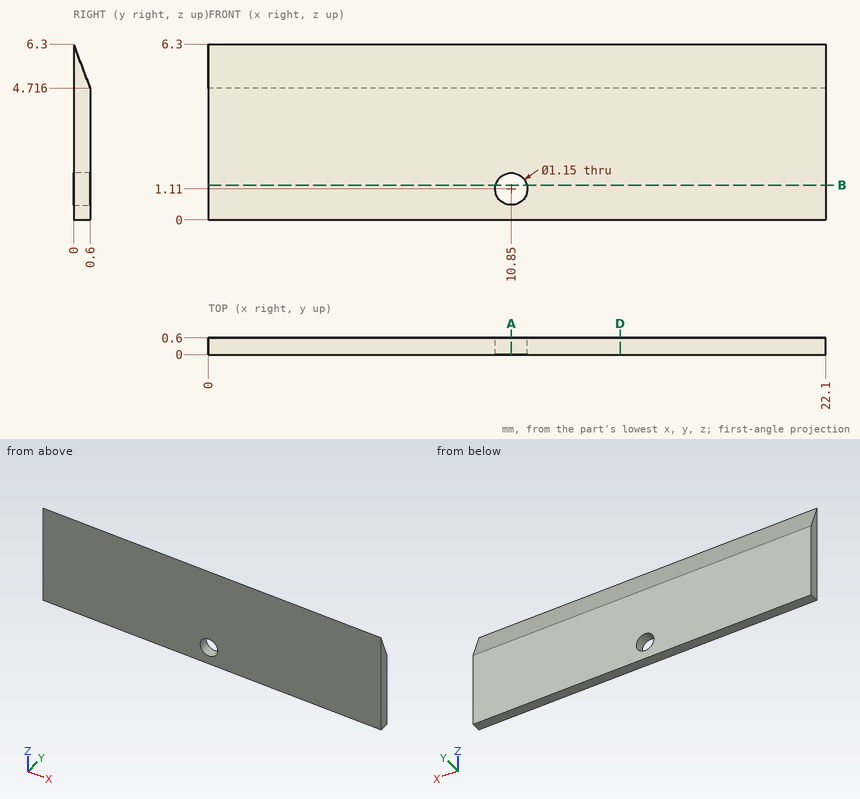
The drawing under review shows one solid part. Ordinate dimensions are in mm from its lowest x, y, z. Round coordinates to 2 decimals unless told otherwise and drop trailing zeros. Loops run counter-clockwise (first coordinate to the right, second up) from the corner with the lowest first, then second, coordinate; pieces in that order, holes last. Notation, with made-up numbers: (-16, 45) - (1, 45) arc R25 cw to (1, 64) - close; hole circle Ø9 at (79, 1.25). An arc over 180 degrees is marked (long way). One line per question, with ' | ' between items.
Q1. Take a section at D-D (x = 14.75). Give the boundary of the cut face in (y, z) (1 decimal).
Taken from the geometry:
outline: (0, 0) - (0.6, 0) - (0.6, 4.7) - (0, 6.3) - close
Q2. Take a section at A-A (x = 10.85). Give the boundary of the cut face in (y, z) (1 decimal).
Taken from the geometry:
outline: (0, 0) - (0.6, 0) - (0.6, 0.5) - (0, 0.5) - close; (0, 1.7) - (0.6, 1.7) - (0.6, 4.7) - (0, 6.3) - close
Q3. For line 1 along X through (y, z) = (0.1, 1) (1 decimal); line 2 along Y through (x, z) = (20.75, 4.75); line 3 along Y through (x, z) = (21, 5.5), list the stretches that pass through material, from the lowest coordinate up. Write a range as [from, to].
Taken from the geometry:
line 1: x = [0, 10.3], [11.4, 22.1] | line 2: y = [0, 0.59] | line 3: y = [0, 0.3]
Q4. Take a section at B-B (z = 1.25). Give the boundary of the cut face in (x, y).
Taken from the geometry:
outline: (0, 0) - (10.29, 0) - (10.29, 0.6) - (0, 0.6) - close; (11.41, 0) - (22.1, 0) - (22.1, 0.6) - (11.41, 0.6) - close
